CAD build for the part. Positions are in the model's coordinates, mm. A direction names the side the tool comes from. Round coordinates to 2 decimals unless told otherwise and drop trailing zeros. Order: outer loops, then holes, each group sorted by start corner. A loop starts at its lowest first (then second) coordinate and runs counter-clockwise, first axis right, second up. Notation, with made-up numbers: (-24, -14.75) -> (-9, -14.75) arc R17 ccw to (-9, -2.75) -> close; hole circle Ø5 at (70.25, -18). An arc over 180 degrees is marked (long way). Return JSON: item names as keys, results as strings. Group by question number.
Q1. Cut at C-C (y = -0.5). Write the cut outline in (x, z).
Q2. Which spindle directions (+Z, -Z, +X, -X, +Y, -Y) get a long thin tool onto all of the face, cutting with end or side? Do faces 1 (the flat face through (20, 0, 1)), 2 (the flat face through (0, 0, 1)). Say none if no direction does.
Q3. Cut at A-A (x = -9). Write the cut outline in (y, z), then the cut area to 3 significant figures.
Q4. Mould opens along Y. For faces 3 (the flat face through (-15, -1.5, 1)), 4 (the flat face through (-30, 4, 1)), 5 (the flat face through (-5, 6.5, 1)) say: +Y half, -Y half, draft (parallel to the pull), parting line (faces both ways), or undercut.
Q5. Cut at B-B (z = 1.55). Write the cut outline in (x, y).
Q6. Probe line 1 along Y through (x, z) = (-21.5, 0.9); line 2 along X through (y, z) = (1, 0.9); line 3 along X through (y, z) = (6.25, 2.1). List the from-to ranges inside material, lowest first.
Q7. Flat gauge pin, fed straight in: pin 1 (0.9 mm diameter, centred on y = 0, z = 1.5, fed in from -X). Where does the tip first touch, or does it go through?
from build123d import *

# Parameters (mm, degrees)
SALIENTE_EXTRUIR1_DEPTH = 3


with BuildPart() as part:
    # Croquis1 → Saliente-Extruir1 (new body)
    with BuildSketch(Plane.XY):
        with BuildLine():
            Line((-29.5, 1.5), (0, 1.5))
            Line((0, 1.5), (0, -1.5))
            Line((0, -1.5), (-29.5, -1.5))
            ThreePointArc((-29.5, -1.5), (-29.853553391, -1.646446609), (-30, -2))
            Line((-30, -2), (-30, -6))
            ThreePointArc((-30, -6), (-29.853553391, -6.353553391), (-29.5, -6.5))
            Line((-29.5, -6.5), (19.5, -6.5))
            ThreePointArc((19.5, -6.5), (19.853553391, -6.353553391), (20, -6))
            Line((20, -6), (20, 0))
            Line((20, 0), (20, 6))
            ThreePointArc((20, 6), (19.853553391, 6.353553391), (19.5, 6.5))
            Line((19.5, 6.5), (-29.5, 6.5))
            ThreePointArc((-29.5, 6.5), (-29.853553391, 6.353553391), (-30, 6))
            Line((-30, 6), (-30, 2))
            ThreePointArc((-30, 2), (-29.853553391, 1.646446609), (-29.5, 1.5))
        make_face()
    extrude(amount=SALIENTE_EXTRUIR1_DEPTH)


solid = part.part
Solution:
{
 "1": {"outline": "(0, 0) -> (20, 0) -> (20, 3) -> (0, 3) -> close"},
 "2": {"face 1": "+Z, -Z, +X, +Y, -Y", "face 2": "+Z, -Z, -X"},
 "3": {"outline": "(-6.5, 0) -> (-1.5, 0) -> (-1.5, 3) -> (-6.5, 3) -> close; (1.5, 0) -> (6.5, 0) -> (6.5, 3) -> (1.5, 3) -> close", "area": "30.0 mm²"},
 "4": {"face 3": "undercut", "face 4": "draft", "face 5": "+Y half"},
 "5": {"outline": "(-30, -6) arc R0.5 ccw to (-29.5, -6.5) -> (19.5, -6.5) arc R0.5 ccw to (20, -6) -> (20, 6) arc R0.5 ccw to (19.5, 6.5) -> (-29.5, 6.5) arc R0.5 ccw to (-30, 6) -> (-30, 2) arc R0.5 ccw to (-29.5, 1.5) -> (0, 1.5) -> (0, -1.5) -> (-29.5, -1.5) arc R0.5 ccw to (-30, -2) -> close"},
 "6": {"line 1": "y = -6.5 to -1.5, 1.5 to 6.5", "line 2": "x = 0 to 20", "line 3": "x = -29.93 to 19.93"},
 "7": {"pin 1": "stops at x = 0"}
}
